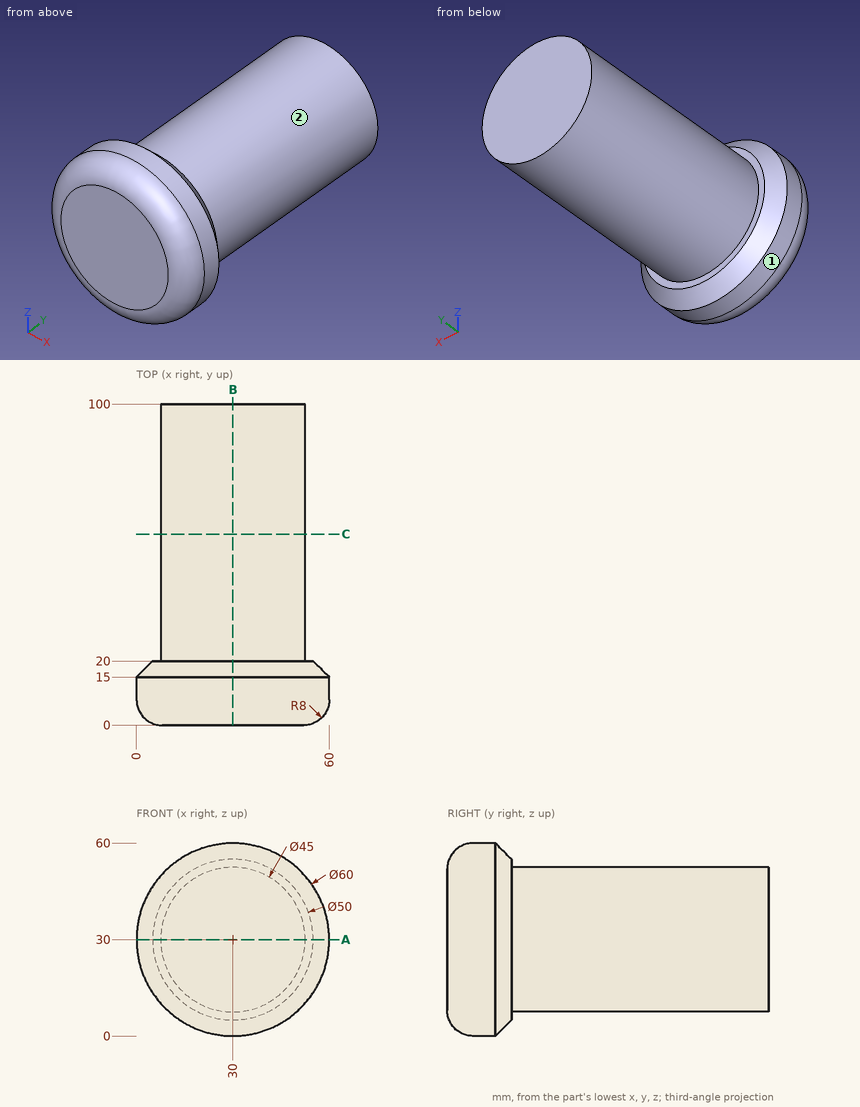
Drawing for the job (mm, zero at the part's lowest x, y, z). A direction names the side the tool comes from. Give positions to 0.01 mm unless a question says otherwise; leave off trailing zeros. Order: outer loops, then holes, each group sorted by start corner. A loop starts at its lowest first (then second) coordinate and runs counter-clockwise, first axis right, second up. Notation, with made-up numbers: (35, 4.5) - (76, 4.5) arc R24 cw to (76, 28.5) - close; hole circle Ø9 at (42, 42). An arc over 180 degrees is marked (long way). Write item = value, one per line. Start each with the question number.
1. Probe line 1 along Z through (x, y) = (44, 46); line 2 along Z through (x, y) = (24.5, 6); line 3 along X through (y, z) = (46.5, 35). List the from-to ranges inside material, lowest first.
2. Cut at B-B, the plane x = 30. List the corners of the cut face in (y, z).
3. Cut at A-A, the plane z = 30. List the corners of the cut face in (x, y), and give its area (3 significant figures).
4. Drop flat-ended pins along their axis: P1, Ø10, axis at y = 39.5, z = 38, coming from the +X side; P2, Ø3, axis at x = 24.5, y = 46, coming from the -Z side; P3, Ø4, axis at y = 16.5, z = 44.5, coming from the +X side. Give the stop position or say it passes through.
5. Which spindle directions (+Z, -Z, +X, -X, +Y, -Y) get a long thin tool onto all of the face, cutting with end or side? Do the marked faces 1 and 2. Say none if no direction does.
6. Cut at C-C, the plane y = 59.5. List the corners of the cut face in (x, z).
Taken from the geometry:
q1.line_1 = 12.39 to 47.61
q1.line_2 = 0.77 to 59.23
q1.line_3 = 8.06 to 51.94
q2.outline = (0, 8) arc R8 ccw to (8, 0) - (15, 0) - (20, 5) - (20, 7.5) - (100, 7.5) - (100, 52.5) - (20, 52.5) - (20, 55) - (15, 60) - (8, 60) arc R8 ccw to (0, 52) - close
q3.outline = (0, 8) arc R8 ccw to (8, 0) - (52, 0) arc R8 ccw to (60, 8) - (60, 15) - (55, 20) - (52.5, 20) - (52.5, 100) - (7.5, 100) - (7.5, 20) - (5, 20) - (0, 15) - close
q3.area = 4,750 mm²
q4.P1 = 52.3
q4.P2 = 7.86
q4.P3 = 56.95
q5.face_1 = +Y, -Y
q5.face_2 = +Y
q6.outline = circle Ø45 at (30, 30)
